```python
from build123d import *

# Parameters (mm, degrees)
SKETCH_W        = 7
SKETCH_H        = 15.401475
PAD_DEPTH       = 10
SKETCH001_W     = 5.211703
SKETCH001_H     = 13.401846
POCKET_DEPTH    = 7
SKETCH002_R     = 0.775886
POCKET001_DEPTH = 7.001
SKETCH003_R     = 0.475645
SKETCH003_R_2   = 1.257083
POCKET002_DEPTH = 10.001
POCKET003_DEPTH = 1


with BuildPart() as part:
    # Sketch → Pad (new body)
    with BuildSketch(Plane.YZ):
        with Locations((-0.5, -1.299263)):
            Rectangle(SKETCH_W, SKETCH_H)
    extrude(amount=PAD_DEPTH)

    # Sketch001 (on Face6 of Pad) → Pocket (cut)
    with BuildSketch(Plane.YZ.offset(10)):
        with Locations((-0.394149, -1.299077)):
            Rectangle(SKETCH001_W, SKETCH001_H)
    extrude(amount=-POCKET_DEPTH, mode=Mode.SUBTRACT)

    # Sketch002 (on Face2 of Pocket) → Pocket001 (cut, through all)
    with BuildSketch(Plane(origin=(0, -4, 0), x_dir=(0, 0, -1), z_dir=(0, -1, 0))):
        with Locations((0.232735, 5.367224)):
            Circle(SKETCH002_R)
    extrude(amount=-POCKET001_DEPTH, mode=Mode.SUBTRACT)

    # Sketch003 (on Face4 of Pocket001) → Pocket002 (cut, through all)
    with BuildSketch(Plane(origin=(0, 0, 0), x_dir=(0, 1, 0), z_dir=(-1, 0, 0))):
        with Locations((-0.756336, 6)):
            Circle(SKETCH003_R)
        with Locations((-1, -3.238254)):
            Circle(SKETCH003_R_2)
    extrude(amount=-POCKET002_DEPTH, mode=Mode.SUBTRACT)

    # Sketch004 (on Face4 of Pocket002) → Pocket003 (cut)
    with BuildSketch(Plane(origin=(0, 0, 0), x_dir=(0, 1, 0), z_dir=(-1, 0, 0))):
        Polygon((-2, 7), (0, 7), (1, 5.745577), (0, 4.55371), (-1.792042, 4.361475), (-3, 5.668684), align=None)
        Polygon((-2, -1), (0, -1), (1.399085, -2.289909), (0.245664, -3.520222), (-2, -3.520222), (-3, -2.289909), align=None)
    extrude(amount=-POCKET003_DEPTH, mode=Mode.SUBTRACT)


solid = part.part
```
For this review, take the finished solid that the model builds, in its own axes (mm). A direction names the side the tool comes from. Round coordinates to 2 decimals unless told otherwise and drop trailing zeros. Loops run counter-clockwise (first coordinate to the right, second up) from the corner with the lowest first, then second, coordinate; pieces in that order, holes last.
(1) We need section C-C (z = -6). Give the boundary of the cut face in (x, y), plus the area to 3 significant figures.
Returned:
outline: (0, -4) - (10, -4) - (10, -3) - (3, -3) - (3, -1.23) - (1, -1.23) - (1, -2.75) - (0, -2.75) - close; (0, 0.8) - (1, 0.8) - (1, -0.28) - (3, -0.28) - (3, 2.21) - (10, 2.21) - (10, 3) - (0, 3) - close
area: 28.1 mm2
(2) We need section B-B (x = 5.75). Give the boundary of the cut face in (y, z), plus the area to 4 significant figures.
Returned:
outline: (-4, -9) - (3, -9) - (3, -0.91) - (2.21, -0.91) - (2.21, -8) - (-3, -8) - (-3, -0.91) - (-4, -0.91) - close; (-4, 0.44) - (-3, 0.44) - (-3, 5.4) - (2.21, 5.4) - (2.21, 0.44) - (3, 0.44) - (3, 6.4) - (-4, 6.4) - close
area: 35.55 mm2
(3) Mouldability with a two-part tool opening along Z and no side actions: class faces 4 (the flat face through (10, 2.6, -1.2)), 5 (the flat face through (7, 0, -8)), 6 (the flat face through (5, -1, -9)) as released by +Z, released by -Z, zero draft, split by the parting line, or undercut.
Returned:
face 4: zero draft
face 5: undercut
face 6: released by -Z
(4) We need section D-D (y = -1.5). Give the boundary of the cut face in (x, z), plus the area to 3 significant figures.
Returned:
outline: (0, -9) - (10, -9) - (10, -8) - (3, -8) - (3, 2.08) - (1, 2.08) - (1, 1) - (0, 1) - (0, -4.39) - (1, -4.39) - (1, -7) - (0, -7) - close; (0, 4.39) - (3, 4.39) - (3, 5.4) - (10, 5.4) - (10, 6.4) - (0, 6.4) - close
area: 49.6 mm2
(5) Clearance check with flat-ended pins moving along their axes: P1, Ø1.3, axis at y = -1.5, z = 2.5, coming from the -X side; P2, Ø2.5, axis at y = -1.5, z = -1.5, coming from the +X side. State where each tip first meets the part, or that it passes through.
Returned:
P1: stops at x = 1
P2: stops at x = 3
(6) Wall thickness on line 1 along Y through (x, z) = (4.5, 3.75); line 2 along Z through (x, y) = (3.5, 0.25); line 3 along Z through (x, y) = (0.75, -2.75): over which ranges is each line inside the solid? List them lowest first.
Returned:
line 1: y = -4 to -3, 2.21 to 3
line 2: z = -9 to -8, 5.4 to 6.4
line 3: z = -9 to -6, -5.4 to 1.97, 2.6 to 6.4
(7) We need section A-A (x = 4.25). Give the boundary of the cut face in (y, z), plus the area to 3 significant figures.
Returned:
outline: (-4, -9) - (3, -9) - (3, 6.4) - (-4, 6.4) - close; hole (-3, -8) - (2.21, -8) - (2.21, 5.4) - (-3, 5.4) - close
area: 38.0 mm2
(8) Tool access review of faces 1 (the flat face through (0.49, -0.88, -4.46)), 2 (the flat face through (4.9, 3, -1.4)), 3 (the flat face through (3, 0, -1)): name each direction out of +Z, -Z, +X, -X, +Y, -Y from which nothing blocks a thin tool from reaching the whole face with its end or side.
Returned:
face 1: -X
face 2: +Z, -Z, +X, -X, +Y
face 3: +X
